Could you check a few things on this model? Use its own coordinates, in mm. Coordinates: 2 decimals unless noted, no trailing zeros. Write each loop counter-clockwise with the first axis right and the second up, starting at its lowest first coordinate (ties: lowest second). Pieces come first, ordered by that corner, then holes. Notation, with made-up numbers: (-11, 70.25) - (38, 70.25) arc R9 cw to (38, 82.25) - close; hole circle Ø6 at (0, -9). An arc over 180 degrees is marked (long way). Answer as a JSON object with one key per item and string values. Group by question number.
1) If we section it at B-B (z = 20.5): Write out the boundary of the cut face in (x, y).
2) If we section it at C-C (z = 2.75): State how many separate pieces and enclosed holes the cut face has, plus the area to 3 significant figures.
3) Will these pins go through, and if not, where does the flat tip stop? pin 1 Ø10 at (x, y) = (26.5, 12.5) entering from +Z; pin 2 Ø1.5 at (x, z) = (39, 17) entering from +Y.
4) We'd pull the mould along X, two halves only. Please class faces 1 (the cylindrical face through (9.73, 11.07, 7.8)), 2 (the flat face through (25, 25, 5)), 3 (the flat face through (50, 10, 10)): released by +X, released by -X, zero draft, split by the parting line, or undercut.
5) Please list where these lines run through material, in increasing order: line 1 along Y through (x, z) = (35.5, 9.5); line 2 along Z through (x, y) = (34.5, 12.25); line 3 along Y through (x, z) = (10, 5.25).
6) If we section it at A-A (x = 20): Write out the boundary of the cut face in (y, z), plus the area to 3 significant figures.
```python
from build123d import *

# Parameters (mm, degrees)
F0_W     = 50
F0_H     = 25
F1_DEPTH = 25
F2_SIZE  = 15
F4_D     = 4.2
F5_SIZE  = 1


with BuildPart() as f1:
    # F0 (on Top) → F1 (new body)
    with BuildSketch(Plane.XY):
        with Locations((25, 12.5)):
            Rectangle(F0_W, F0_H)
    extrude(amount=F1_DEPTH)

    # F2
    f2_edges = [f1.edges().sort_by_distance(p)[0] for p in [
        (25, 25, 25),
    ]]
    chamfer(f2_edges, length=F2_SIZE)

    # F4 (through all)
    with Locations(Plane(origin=(0, 17.5, 17.5), x_dir=(-1, 0, 0), z_dir=(0, 0.7071067812, 0.7071067812))):
        with Locations((-10, -4.3933982822), (-35, -4.3933982822)):
            Hole(F4_D / 2)

    # F5
    f5_edges = [f1.edges().sort_by_distance(p)[0] for p in [
        (25, 25, 0),
    ]]
    chamfer(f5_edges, length=F5_SIZE)


solid = f1.part
```
Here are the results:
{
 "1": {"outline": "(0, 0) - (50, 0) - (50, 14.5) - (0, 14.5) - close"},
 "2": {"separate pieces": "1", "enclosed holes": "2", "area": "1,210 mm²"},
 "3": {"pin 1": "stops at z = 25", "pin 2": "stops at y = 18.75"},
 "4": {"face 1": "undercut", "face 2": "zero draft", "face 3": "released by +X"},
 "5": {"line 1": "y = 0 to 12.83, 18.6 to 25", "line 2": "z = 0 to 3.15, 8.92 to 22.75", "line 3": "y = 0 to 8.49, 14.43 to 25"},
 "6": {"outline": "(0, 0) - (24, 0) - (25, 1) - (25, 10) - (10, 25) - (0, 25) - close", "area": "512 mm²"}
}
